```python
from build123d import *

# Parameters (mm, degrees)
SKETCH1_R           = 3.683
BASE_EXTRUDE_DEPTH  = 3.937
SKETCH2_R           = 2.3876
CUT_EXTRUDE1_DEPTH  = 7.529084698
CUT_EXTRUDE2_DEPTH  = 0.762
CIRPATTERN1_COUNT   = 16
BOSS_EXTRUDE1_DEPTH = 3.175
FILLET1_R           = 0.396875
FILLET2_R           = 0.1984375


with BuildPart() as part:
    # Sketch1 → Base-Extrude (new body)
    with BuildSketch(Plane(origin=(0, 0, 0), x_dir=(1, 0, 0), z_dir=(0, 1, 0))):
        with Locations(Location((0, 0, 0), (0, 0, 270))):
            Circle(SKETCH1_R)
    extrude(amount=BASE_EXTRUDE_DEPTH)

    # Sketch2 → Cut-Extrude1 (cut, through all)
    with BuildSketch(Plane(origin=(0, 3.937, 0), x_dir=(-1, 0, 0), z_dir=(0, 1, 0))):
        with Locations(Location((0, 0, 0), (0, 0, 90))):
            Circle(SKETCH2_R)
    extrude(amount=-CUT_EXTRUDE1_DEPTH, mode=Mode.SUBTRACT)

    # Sketch4 → Cut-Revolve1 (revolve, cut)
    with BuildSketch(Plane.XY, mode=Mode.PRIVATE) as cut_revolve1_sk:
        with BuildLine():
            Line((3.683, 2.921), (3.038418755, 2.529768267))
            ThreePointArc((3.038418755, 2.529768267), (2.794, 2.0955), (3.038418755, 1.661231733))
            Line((3.038418755, 1.661231733), (3.683, 1.27))
            Line((3.683, 1.27), (3.683, 2.921))
        make_face()
    revolve(cut_revolve1_sk.sketch.rotate(Axis((0, 0, 0), (0, 1, 0)), 90), axis=Axis((0, 0, 0), (0, 1, 0)), mode=Mode.SUBTRACT)

    # Sketch5 → Cut-Extrude2 (cut)
    with BuildSketch(Plane(origin=(16.494267977, 0, 2.582932293), x_dir=(1, 0, 0), z_dir=(0, -1, 0))):
        with BuildLine():
            Line((-18.872782439, -2.374839241), (-20.163253051, -2.261937692))
            ThreePointArc((-20.163253051, -2.261937692), (-20.177267977, -2.582932293), (-20.163253051, -2.903926893))
            Line((-20.163253051, -2.903926893), (-18.872782439, -2.791025344))
            ThreePointArc((-18.872782439, -2.791025344), (-18.881867977, -2.582932293), (-18.872782439, -2.374839241))
        make_face()
    cut_extrude2 = extrude(amount=-CUT_EXTRUDE2_DEPTH, mode=Mode.SUBTRACT)

    # CirPattern1: Cut-Extrude2 ×16 about axis
    cirpattern1_axis = Axis((0, 0, 0), (0, 1, 0))
    for i in range(1, CIRPATTERN1_COUNT):
        add(cut_extrude2.rotate(cirpattern1_axis, i * 360 / CIRPATTERN1_COUNT), mode=Mode.SUBTRACT)

    # Sketch6 → Boss-Extrude1 (add)
    with BuildSketch(Plane(origin=(0, 3.937, 0), x_dir=(-1, 0, 0), z_dir=(0, 1, 0))):
        with BuildLine():
            Line((-0.92075, -2.202919244), (-0.92075, -0.92075))
            Line((-0.92075, -0.92075), (-2.202919244, -0.92075))
            ThreePointArc((-2.202919244, -0.92075), (-1.688288151, -1.688288151), (-0.92075, -2.202919244))
        make_face()
        with BuildLine():
            Line((2.202919244, 0.92075), (0.92075, 0.92075))
            Line((0.92075, 0.92075), (0.92075, 2.202919244))
            ThreePointArc((0.92075, 2.202919244), (1.688288151, 1.688288151), (2.202919244, 0.92075))
        make_face()
    extrude(amount=-BOSS_EXTRUDE1_DEPTH)

    # Fillet1
    fillet1_edges = [part.edges().sort_by_distance(p)[0] for p in [
        (0.92075, 2.3495, -0.92075),
        (-0.92075, 2.3495, 0.92075),
    ]]
    fillet(fillet1_edges, radius=FILLET1_R)

    # Fillet2
    fillet2_edges = [part.edges().sort_by_distance(p)[0] for p in [
        (-3.683, 2.921, 0),
        (-3.683, 2.921, 0),
    ]]
    fillet(fillet2_edges, radius=FILLET2_R)


solid = part.part
```
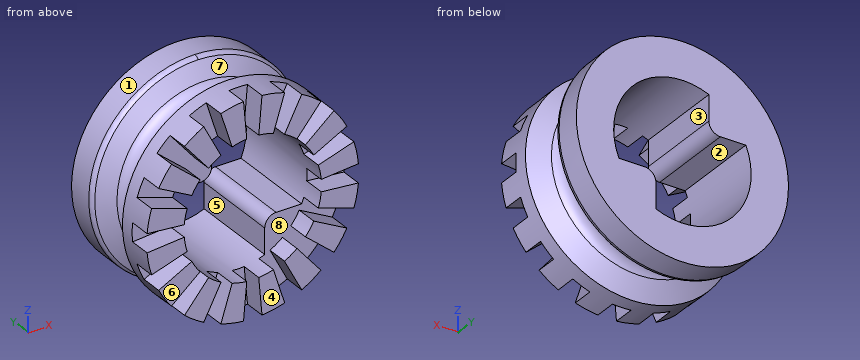
Model file for the job. Use its own axes, mm. Face numbers are marked on the shaded views. A direction names the side the tool comes from. Give positions to 0.01 mm unless a question says otherwise; leave off trailing zeros. Order: outer loops, then holes, each group sorted by start corner. A loop starts at its lowest first (then second) coordinate and runs counter-clockwise, first axis right, second up.
1) Mould opens along X. For the marked faces 1, 2, 3 and 4 say: +X half, -X half, draft (parallel to the pull), parting line (faces both ways), or undercut.
2) Wall check: probe 1 along X at (y, z) = (3.7, 0); probe 2 along X at (y, z) = (2.9, 1.5); probe 3 along Z at (x, y) = (-1.25, 3.65). Give the ranges that are in metal, low to high.
3) 3-axis set-ups, long thin cutter, end or side, ignore diameter. For the marked faces 5, 6, 7 and 8: which of +Z, -Z, +X, -X, +Y, -Y reach the whole face in a straight line?
4) Pin check, flat tip, straight feed: pin 1 (1 mm diameter, centred on x = -2, y = 2, fed in from -Z). Stop position of the tip, or through.
5) Saw through at B-B, the plane y = 2.05. Write the cut outline in (x, z), then the cut area to 3 significant figures.
6) Saw through at A-A, the plane y = 1. Write the cut outline in (x, z), then the cut area to 3 significant figures.
Computed:
1. face 1: parting line
1. face 2: undercut
1. face 3: undercut
1. face 4: draft
2. probe 1: x = -3.68 to -2.39, 2.39 to 3.68
2. probe 2: x = -3.31 to -0.92, 1.86 to 3.31
2. probe 3: z = -3.46 to -2.03, 0.93 to 3.46
3. face 5: +Y, -Y
3. face 6: +Z, -Z, +X, -X, -Y
3. face 7: none
3. face 8: -Y
4. pin 1: stops at z = -2.69
5. outline: circle Ø5.59 at (0, 0); hole (-2.2, 0.92) arc R2.39 ccw to (0.92, -2.2) - (0.92, -1.32) arc R0.4 cw to (1.32, -0.92) - (2.2, -0.92) arc R2.39 ccw to (-0.92, 2.2) - (-0.92, 1.32) arc R0.4 cw to (-1.32, 0.92) - close
5. area: 8.66 mm2
6. outline: circle Ø7.37 at (0, 0); hole (-2.2, 0.92) arc R2.39 ccw to (0.92, -2.2) - (0.92, -1.32) arc R0.4 cw to (1.32, -0.92) - (2.2, -0.92) arc R2.39 ccw to (-0.92, 2.2) - (-0.92, 1.32) arc R0.4 cw to (-1.32, 0.92) - close
6. area: 26.7 mm2
